Source: three-view drawing plus pictorial views. Frame: mm from the lowest corner of the part. Give positions to 0.01 mm unless a question says otherwise; leave off trailing zeros. Loops run counter-clockwise (first coordinate to the right, second up) from the corner with the lowest first, then second, coordinate; pieces in that order, holes last. Notation, with made-up numbers: (-31, 54.25) - (10, 54.25) arc R20 cw to (10, 61.25) - close; hole circle Ø1 at (50.5, 13). An arc over 180 degrees is marked (long way). One line per item, written item: value.
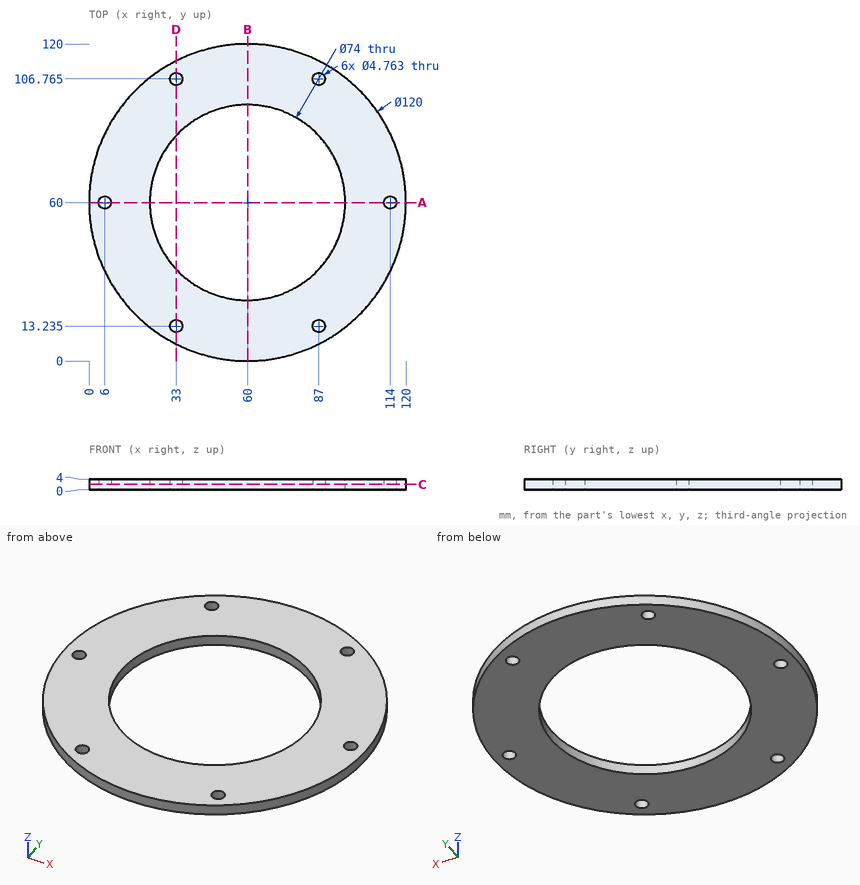
Item 1: Section D-D, the plane x = 33. Output: boundary loops of the cut face in (y, z) (1 decimal).
Verdict:
outline: (6.4, 0) - (10.9, 0) - (10.9, 4) - (6.4, 4) - close; (15.6, 0) - (34.7, 0) - (34.7, 4) - (15.6, 4) - close; (85.3, 0) - (104.4, 0) - (104.4, 4) - (85.3, 4) - close; (109.1, 0) - (113.6, 0) - (113.6, 4) - (109.1, 4) - close
Item 2: Section C-C, the plane z = 1.95. Output: boundary loops of the cut face in (x, y) (1 decimal), and give its area (3 significant figures).
Verdict:
outline: circle Ø120 at (60, 60); hole circle Ø4.8 at (6, 60); hole circle Ø74 at (60, 60); hole circle Ø4.8 at (33, 13.2); hole circle Ø4.8 at (33, 106.8); hole circle Ø4.8 at (87, 13.2); hole circle Ø4.8 at (87, 106.8); hole circle Ø4.8 at (114, 60)
area: 6,900 mm^2
Item 3: Pin query (flat end, axial travel): P1, Ø1, axis at x = 82.5, z = 0.5, coming from the -Y side; P2, Ø1, axis at x = 33, z = 3.5, coming from the +Y side; P3, Ø4.5, axis at x = 87, y = 106.77, coming from the +Z side (3 decimals); P4, Ø1.5, axis at x = 86, z = 1.5, coming from the -Y side. Return the tip coordinate at first contact, or that it passes through.
Verdict:
P1: stops at y = 4.18
P2: stops at y = 113.83
P3: passes through
P4: stops at y = 5.57
Item 4: Section A-A, the plane y = 60. Output: boundary loops of the cut face in (x, z).
Verdict:
outline: (0, 0) - (3.62, 0) - (3.62, 4) - (0, 4) - close; (8.38, 0) - (23, 0) - (23, 4) - (8.38, 4) - close; (97, 0) - (111.62, 0) - (111.62, 4) - (97, 4) - close; (116.38, 0) - (120, 0) - (120, 4) - (116.38, 4) - close
Item 5: Material intervals for L1, parallel to Y at x = 33, z = 3.05 (1 decimal); L2, parallel to Y at x = 60, z = 1.15; L3, parallel to Y at x = 27, z = 1.35 (1 decimal), sorted ascending.
Verdict:
L1: y = 6.4 to 10.9, 15.6 to 34.7, 85.3 to 104.4, 109.1 to 113.6
L2: y = 0 to 23, 97 to 120
L3: y = 9.9 to 43.3, 76.7 to 110.1
Item 6: Section B-B, the plane x = 60. Output: boundary loops of the cut face in (y, z), and give its area (3 significant figures).
Verdict:
outline: (0, 0) - (23, 0) - (23, 4) - (0, 4) - close; (97, 0) - (120, 0) - (120, 4) - (97, 4) - close
area: 184 mm^2
